Geometry: final body of the model. Coordinates: model frame, mm. Face numbers are marked on the shaded views. Coordinates: 2 decimals unless noted, no trailing zeros. Order: outer loops, then holes, each group sorted by start corner. A loop starts at its lowest first (then second) coordinate and runs counter-clockwise, first axis right, second up. Notation, with made-up numbers: (66, 36) - (125, 36) arc R12 cw to (125, 49) - close; hole circle Ø2 at (86.25, -34). An arc over 180 degrees is marked (long way). Use one line per item in the form item = value. Start each with the question number.
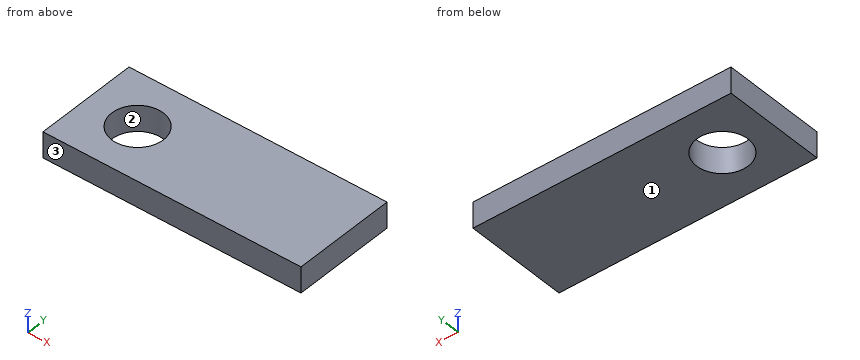
```python
from build123d import *

# Parameters (mm, degrees)
F0_W     = 100
F0_H     = 40
F0_R     = 10
F1_DEPTH = 10


with BuildPart() as f1:
    # F0 (on Top) → F1 (new body)
    with BuildSketch(Plane.XY):
        with Locations((-46.849999, 35.900001)):
            Rectangle(F0_W, F0_H)
        with Locations((-76.849999, 35.900001)):
            Circle(F0_R, mode=Mode.SUBTRACT)
    extrude(amount=-F1_DEPTH)


solid = f1.part
```
(1) Material intervals for L1, parallel to Y at x = -76.85, z = -7.5; L2, parallel to X at y = 27.5, z = -7.75; L3, parallel to Y at x = -83.5, z = -7.5, sorted ascending. Write a range as from..to.
(2) Cut plane C-C on z = -8.25. Return the cut outline in (x, y).
(3) Draft query along Y for the marked faces 1, 2 and 3. Return one class per face: released by +Y, released by -Y, zero draft, split by the parting line, or undercut.
(4) Cut plane B-B on y = 42. Return the cut outline in (x, z).
(5) Contact query for a flat-ended pin moving along its axis: pin 1 Ø5 at (x, y) = (-40.5, 25) entering from +Z. Output: stop coordinate, or through.
(6) Cut plane A-A on x = -76.85. Return the cut outline in (y, z).
Check sheet entries:
q1.L1 = 15.9..25.9, 45.9..55.9
q1.L2 = -96.85..-82.28, -71.42..3.15
q1.L3 = 15.9..28.43, 43.37..55.9
q2.outline = (-96.85, 15.9) - (3.15, 15.9) - (3.15, 55.9) - (-96.85, 55.9) - close; hole circle Ø20 at (-76.85, 35.9)
q3.face_1 = zero draft
q3.face_2 = undercut
q3.face_3 = released by -Y
q4.outline = (-96.85, -10) - (-84.77, -10) - (-84.77, 0) - (-96.85, 0) - close; (-68.93, -10) - (3.15, -10) - (3.15, 0) - (-68.93, 0) - close
q5.pin_1 = 0
q6.outline = (15.9, -10) - (25.9, -10) - (25.9, 0) - (15.9, 0) - close; (45.9, -10) - (55.9, -10) - (55.9, 0) - (45.9, 0) - close
